Model file for the job. Use its own axes, mm. A direction names the side the tool comes from. Give positions to 0.01 mm unless a question says otherwise; leave off trailing zeros. Loops run counter-clockwise (first coordinate to the right, second up) from the corner with the lowest first, then second, coordinate; pieces in that order, holes last. Notation, with made-up numbers: M 77.25,14.5 L 125.25,14.5 A19 cw 125.25,37.5 Z; hole C 8.5,69.25 d6. An arc over 180 degrees is marked long. Use CSV: the item, a comma, the result in double quotes. Start each with the question number.
(1) Wall check: line 1 along X through (y, z) = (0.2, -24.5); line 2 along X through (y, z) = (0.55, 24.5); line 3 along Z through (x, y) = (-55.5, 0.45). Give the ranges that are in metal, low to high. Write a range as from..to.
(2) Slice it at B-B on z = -24.5. List the corners of the cut face in (x, y), and give its area (3 significant figures).
(3) Slice it at C-C on x = -55.5. List the corners of the cut face in (y, z), and give its area (3 significant figures).
(4) Slice it at A-A on y = 2.5. List the corners of the cut face in (x, z), and give its area (3 significant figures).
(5) Flat gauge pins, fed straight in: P1, Ø4.5, axis at x = -8.5, y = 4.5, coming from the -Z side; P2, Ø14.5, axis at x = 18, z = -14, coming from the +Y side; P3, Ø4, axis at x = 21, y = 4.5, coming from the +Z side. Where does each tip first touch, or does it go through?
(6) Two-plate mould, pull along X, no slides. Class faces 6 (the face through (58.7, 0.5, 0.1)), 7 (the face through (52.8, 4, -24.2)), 8 (the face through (57, 1, 26)): pulls with the +X half, pulls with the -X half, needs draft (parallel to the pull), parting line crosses it, or undercut.
(7) Slice it at D-D on z = 24.5. List the corners of the cut face in (x, y), and give its area (3 significant figures).
(8) Tool access for faces 1 (the face through (-52.9, 4, 25.3)), 2 (the face through (-54, 4, -22)), 3 (the face through (51.7, 2, 25)), 4 (the face through (-51.7, 2, -24)), 5 (the face through (-54.16, 2.52, -26.61)): list every direction of +Z, -Z, +X, -X, +Y, -Y with a clear straight run to the whole face (end or side of a thin tool).
```python
from build123d import *

# Parameters (mm, degrees)
SKETCH1_W           = 117.4
SKETCH1_H           = 55.4
BOSS_EXTRUDE1_DEPTH = 1
SKETCH2_W           = 7
SKETCH2_H           = 7
BOSS_EXTRUDE2_DEPTH = 3
SKETCH3_R           = 1.35
CUT_EXTRUDE1_DEPTH  = 5
SKETCH7_W           = 30
SKETCH7_H           = 6
CUT_EXTRUDE5_DEPTH  = 5
SKETCH9_R           = 2.5
CUT_EXTRUDE6_DEPTH  = 3
SKETCH10_W          = 117.4
SKETCH10_H          = 1
BOSS_EXTRUDE3_DEPTH = 9


with BuildPart() as part:
    # Sketch1 → Boss-Extrude1 (new body)
    with BuildSketch(Plane(origin=(0, 0, 0), x_dir=(1, 0, 0), z_dir=(0, 1, 0))):
        Rectangle(SKETCH1_W, SKETCH1_H)
    extrude(amount=BOSS_EXTRUDE1_DEPTH)

    # Sketch2 → Boss-Extrude2 (add)
    with BuildSketch(Plane(origin=(0, 1, 0), x_dir=(1, 0, 0), z_dir=(0, 1, 0))):
        with Locations((55.2, 24.2)):
            Rectangle(SKETCH2_W, SKETCH2_H)
        with Locations((-55.2, 24.2)):
            Rectangle(SKETCH2_W, SKETCH2_H)
        with Locations((55.2, -24.2)):
            Rectangle(SKETCH2_W, SKETCH2_H)
        with Locations((-55.2, -24.2)):
            Rectangle(SKETCH2_W, SKETCH2_H)
    extrude(amount=BOSS_EXTRUDE2_DEPTH)

    # Sketch3 → Cut-Extrude1 (cut, through all)
    with BuildSketch(Plane(origin=(0, 4, 0), x_dir=(1, 0, 0), z_dir=(0, 1, 0))):
        with Locations((-55.5, 24.5)):
            Circle(SKETCH3_R)
        with Locations((55.5, 24.5)):
            Circle(SKETCH3_R)
        with Locations((55.5, -24.5)):
            Circle(SKETCH3_R)
        with Locations((-55.5, -24.5)):
            Circle(SKETCH3_R)
    extrude(amount=-CUT_EXTRUDE1_DEPTH, mode=Mode.SUBTRACT)

    # Sketch7 → Cut-Extrude5 (cut, through all)
    with BuildSketch(Plane.XZ):
        with Locations((36.7, 24.7)):
            Rectangle(SKETCH7_W, SKETCH7_H)
        with Locations((-36.7, 24.7)):
            Rectangle(SKETCH7_W, SKETCH7_H)
    extrude(amount=-CUT_EXTRUDE5_DEPTH, mode=Mode.SUBTRACT)

    # Sketch9 → Cut-Extrude6 (cut)
    with BuildSketch(Plane(origin=(0, 4, 0), x_dir=(1, 0, 0), z_dir=(0, 1, 0))):
        with Locations((-55.5, 24.5)):
            Circle(SKETCH9_R)
        with Locations((55.5, 24.5)):
            Circle(SKETCH9_R)
        with Locations((55.5, -24.5)):
            Circle(SKETCH9_R)
        with Locations((-55.5, -24.5)):
            Circle(SKETCH9_R)
    extrude(amount=-CUT_EXTRUDE6_DEPTH, mode=Mode.SUBTRACT)

    # Sketch10 → Boss-Extrude3 (add)
    with BuildSketch(Plane(origin=(0, 1, 0), x_dir=(1, 0, 0), z_dir=(0, 1, 0))):
        with Locations((0, -21.2)):
            Rectangle(SKETCH10_W, SKETCH10_H)
    extrude(amount=BOSS_EXTRUDE3_DEPTH)


solid = part.part
```
Reply:
1,line 1,"x = -58.7..-56.85, -54.15..54.15, 56.85..58.7"
1,line 2,"x = -58.7..-56.85, -54.15..-51.7, -21.7..21.7, 51.7..54.15, 56.85..58.7"
1,line 3,"z = -27.7..-25.85, -23.15..23.15, 25.85..27.7"
2,outline,"M -58.7,0 L -56.85,0 L -56.85,1 L -58,1 L -58,4 L -58.7,4 Z; M -54.15,0 L 54.15,0 L 54.15,1 L 53,1 L 53,4 L 51.7,4 L 51.7,1 L -51.7,1 L -51.7,4 L -53,4 L -53,1 L -54.15,1 Z; M 56.85,0 L 58.7,0 L 58.7,4 L 58,4 L 58,1 L 56.85,1 Z"
2,area,"124 mm^2"
3,outline,"M 0,-27.7 L 4,-27.7 L 4,-27 L 1,-27 L 1,-25.85 L 0,-25.85 Z; M 0,-23.15 L 1,-23.15 L 1,-22 L 4,-22 L 4,-20.7 L 1,-20.7 L 1,20.7 L 10,20.7 L 10,21.7 L 4,21.7 L 4,22 L 1,22 L 1,23.15 L 0,23.15 Z; M 0,25.85 L 1,25.85 L 1,27 L 4,27 L 4,27.7 L 0,27.7 Z"
3,area,"68.0 mm^2"
4,outline,"M -58.7,-27.7 L -51.7,-27.7 L -51.7,-20.7 L -58.7,-20.7 Z; M -58.7,20.7 L 58.7,20.7 L 58.7,27.7 L 51.7,27.7 L 51.7,21.7 L -51.7,21.7 L -51.7,27.7 L -58.7,27.7 Z; M 51.7,-27.7 L 58.7,-27.7 L 58.7,-20.7 L 51.7,-20.7 Z; hole C -55.5,-24.5 d5; hole C -55.5,24.5 d5; hole C 55.5,-24.5 d5; hole C 55.5,24.5 d5"
4,area,"221 mm^2"
5,P1,"stops at z = 20.7"
5,P2,"stops at y = 1"
5,P3,"stops at z = 21.7"
6,face 6,"pulls with the +X half"
6,face 7,"needs draft"
6,face 8,"undercut"
7,outline,"M -58.7,0 L -56.85,0 L -56.85,1 L -58,1 L -58,4 L -58.7,4 Z; M -54.15,0 L -51.7,0 L -51.7,4 L -53,4 L -53,1 L -54.15,1 Z; M -21.7,0 L 21.7,0 L 21.7,1 L -21.7,1 Z; M 51.7,0 L 54.15,0 L 54.15,1 L 53,1 L 53,4 L 51.7,4 Z; M 56.85,0 L 58.7,0 L 58.7,4 L 58,4 L 58,1 L 56.85,1 Z"
7,area,"64.0 mm^2"
8,face 1,"+Z, +X, -X, +Y"
8,face 2,"-Z, +X, -X, +Y"
8,face 3,"+Z, +Y, -Y"
8,face 4,"-Z, +Y"
8,face 5,"+Y"
